Job drawing, mm, ordinate dimensions from the low corner. One solid piece. Give positions to 0.01 mm unless a question says otherwise; leave off trailing zeros. Loops run counter-clockwise (first coordinate to the right, second up) from the corner with the lowest first, then second, coordinate; pieces in that order, holes last. Notation, with made-up numbers: (34.25, 16) - (52.25, 16) arc R28 cw to (52.25, 54) - close; hole circle Ø5 at (-18.5, 49.5). An arc over 180 degrees is marked (long way). Answer as CSV lines item,"result". Start each with the question number.
Item 1: Drill centre lines: L1, parallel to X at y = 71, z = 3.5; L2, parallel to Y at x = 310, z = 6.25. Where is each one in solid material? Low to high. Write a range as from..to.
Item 2: Saw through at C-C on y = 71.5. Give the cut face in (x, z).
Item 3: Saw through at A-A on z = 13. Give the cut face in (x, y), plus the area to 3 significant figures.
Item 4: Saw through at B-B on x = 114.5. Give the cut face in (y, z), plus the area to 3 significant figures.
Item 5: Pin check, flat tip, straight feed: pin 1 (3 mm diameter, centred on y = 58, z = 8, fed in from -X). Stop position of the tip, or through.
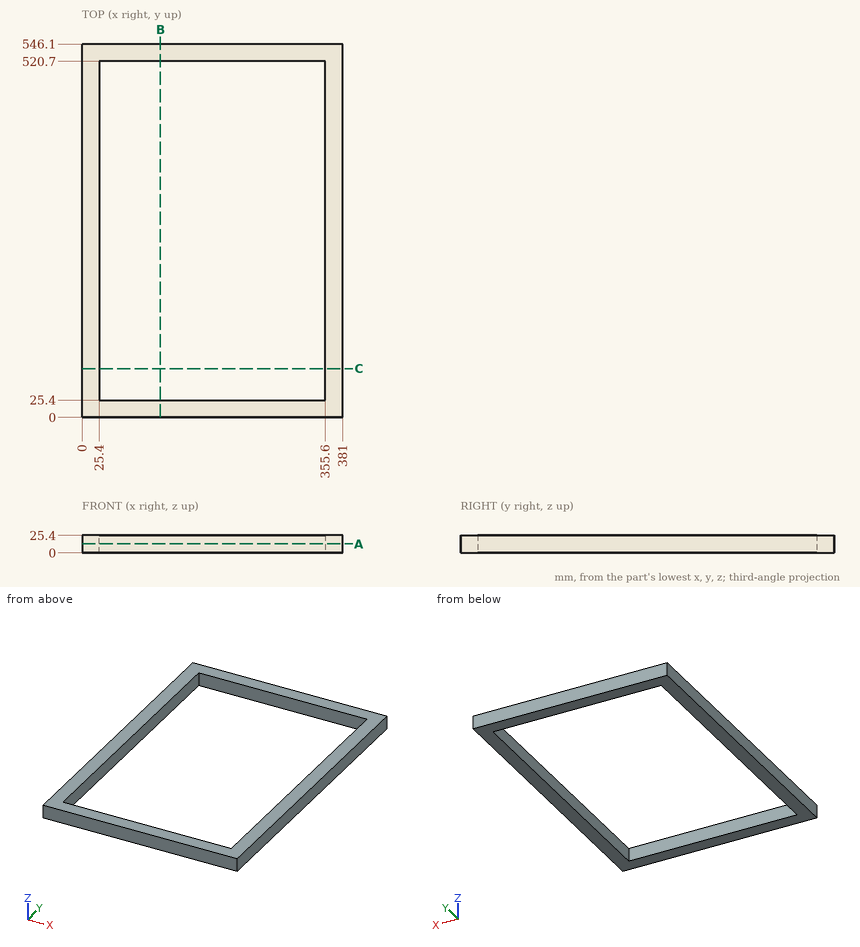
Responses:
1,L1,"0..25.4, 355.6..381"
1,L2,"0..25.4, 520.7..546.1"
2,outline,"(0, 0) - (25.4, 0) - (25.4, 25.4) - (0, 25.4) - close; (355.6, 0) - (381, 0) - (381, 25.4) - (355.6, 25.4) - close"
3,outline,"(0, 0) - (381, 0) - (381, 546.1) - (0, 546.1) - close; hole (25.4, 25.4) - (355.6, 25.4) - (355.6, 520.7) - (25.4, 520.7) - close"
3,area,"44,500 mm2"
4,outline,"(0, 0) - (25.4, 0) - (25.4, 25.4) - (0, 25.4) - close; (520.7, 0) - (546.1, 0) - (546.1, 25.4) - (520.7, 25.4) - close"
4,area,"1,290 mm2"
5,pin 1,"x = 0"
